For this review, take the finished solid that the model builds, in its own axes (mm). A direction names the side the tool comes from. Round coordinates to 2 decimals unless told otherwise and drop trailing zeros. Order: outer loops, then holes, each group sorted by start corner. A loop starts at its lowest first (then second) coordinate and runs counter-clockwise, first axis right, second up. Notation, with made-up numbers: (71.25, -36.75) -> (82.25, -36.75) arc R23 ccw to (82.25, -11.75) -> close; hole circle Ø1 at (31.25, -22.75). An arc over 180 degrees is marked (long way). Use a Markdown table: item, result. Add a question column.
1) Consider section C-C (x = 30). State the section outline as (y, z) points (3 decimals).
2) Consider section A-A (y = -7). State the section outline as (x, z) points (3 decimals), plus the area to 3 significant figures.
3) Clearance check with flat-ended pins moving along their axes: P1, Ø1.6, axis at y = 0.5, z = 11, coming from the +X side; P2, Ø1, axis at y = 1, z = 44, coming from the -X side; P3, Ø4, axis at x = 66.5, y = -5.5, coming from the -Z side (3 decimals). State where each tip first meets the part, or that it passes through.
4) Wall thickness on line 1 along Z through (x, y) = (30, 1) (3 decimals); line 2 along X through (y, z) = (-7.5, 26); line 3 along Y through (x, z) = (14, 24): over which ranges is each line inside the solid? List them lowest first. Write a range as [from, to].
5) Consider section D-D (y = 1). State the section outline as (x, z) points (3 decimals), plus the area to 3 significant figures.
6) Draft analysis for pull direction X (two halves, no side actions). For faces 5 (the face through (63.4, 1, 44)), 6 (the face through (-5, -3, 28)), 7 (the face through (60.4, 1, 45)), 8 (the face through (66, -9, 28)), state which applies: pulls with the +X half, pulls with the -X half, needs draft (parallel to the pull), parting line crosses it, or undercut.
7) Consider section B-B (z = 6). State the section outline as (x, y) points.
8) Machinability: for faces 1 (the face through (39, 0, 29)), 2 (the face through (63.4, 1, 13)), 3 (the face through (31, 1, 3)), 4 (the face through (-3, -3, 31.755)), which of the approach directions +Z, -Z, +X, -X, +Y, -Y give a long, thin tool a straight path to every point of the face, cutting with its end or side? Answer none if there is none.
```python
from build123d import *

# Parameters (mm, degrees)
SKETCH_1_W      = 57.4
SKETCH_1_H      = 19.255
SKETCH_1_H_2    = 21.645
EXTRUDE_1_DEPTH = 2
FILLET_1_R      = 2
SKETCH_2_W      = 4
SKETCH_2_H      = 7.5
EXTRUDE_2_DEPTH = 9


with BuildPart() as part:
    # Эскиз1 → Бобышка-Вытянуть1 (new body)
    with BuildSketch(Plane(origin=(0, 0, 0), x_dir=(1, 0, 0), z_dir=(0, 1, 0))):
        Polygon((63.4, -24.255), (68.4, -24.255), (68.4, -31.755), (63.4, -31.755), (63.4, -58.4), (0, -58.4), (0, -31.755), (-5, -31.755), (-5, -24.255), (0, -24.255), (0, 0), (63.4, 0), align=None)
        with Locations((31.7, -12.6275)):
            Rectangle(SKETCH_1_W, SKETCH_1_H, mode=Mode.SUBTRACT)
        with Locations((31.7, -44.5775)):
            Rectangle(SKETCH_1_W, SKETCH_1_H_2, mode=Mode.SUBTRACT)
    extrude(amount=EXTRUDE_1_DEPTH)

    # Скругление1
    fillet_1_edges = [part.edges().sort_by_distance(p)[0] for p in [
        (0, 1, 0),
        (63.4, 1, 0),
        (63.4, 1, 58.4),
        (0, 1, 58.4),
    ]]
    fillet(fillet_1_edges, radius=FILLET_1_R)

    # Эскиз2 → Бобышка-Вытянуть2 (add)
    with BuildSketch(Plane(origin=(0, 0, 0), x_dir=(-1, 0, 0), z_dir=(0, -1, 0))):
        with Locations((3, -28.005)):
            Rectangle(SKETCH_2_W, SKETCH_2_H)
        with Locations((-66.4, -28.005)):
            Rectangle(SKETCH_2_W, SKETCH_2_H)
    extrude(amount=EXTRUDE_2_DEPTH)


solid = part.part
```
Results list:
| question | item | result |
|---|---|---|
| 1 | outline | (0, 0) -> (2, 0) -> (2, 3) -> (0, 3) -> close; (0, 22.255) -> (2, 22.255) -> (2, 33.755) -> (0, 33.755) -> close; (0, 55.4) -> (2, 55.4) -> (2, 58.4) -> (0, 58.4) -> close |
| 2 | outline | (-5, 24.255) -> (-1, 24.255) -> (-1, 31.755) -> (-5, 31.755) -> close; (64.4, 24.255) -> (68.4, 24.255) -> (68.4, 31.755) -> (64.4, 31.755) -> close |
| 2 | area | 60.0 mm2 |
| 3 | P1 | x = 63.4 |
| 3 | P2 | x = 0 |
| 3 | P3 | z = 24.255 |
| 4 | line 1 | [0, 3], [22.255, 33.755], [55.4, 58.4] |
| 4 | line 2 | [-5, -1], [64.4, 68.4] |
| 4 | line 3 | [0, 2] |
| 5 | outline | (-5, 24.255) -> (0, 24.255) -> (0, 2) arc R2 ccw to (2, 0) -> (61.4, 0) arc R2 ccw to (63.4, 2) -> (63.4, 24.255) -> (68.4, 24.255) -> (68.4, 31.755) -> (63.4, 31.755) -> (63.4, 56.4) arc R2 ccw to (61.4, 58.4) -> (2, 58.4) arc R2 ccw to (0, 56.4) -> (0, 31.755) -> (-5, 31.755) -> close; hole (3, 3) -> (60.4, 3) -> (60.4, 22.255) -> (3, 22.255) -> close; hole (3, 33.755) -> (60.4, 33.755) -> (60.4, 55.4) -> (3, 55.4) -> close |
| 5 | area | 1,430 mm2 |
| 6 | face 5 | pulls with the +X half |
| 6 | face 6 | pulls with the -X half |
| 6 | face 7 | undercut |
| 6 | face 8 | needs draft |
| 7 | outline | (0, 0) -> (3, 0) -> (3, 2) -> (0, 2) -> close; (60.4, 0) -> (63.4, 0) -> (63.4, 2) -> (60.4, 2) -> close |
| 8 | face 1 | +Z, -Z, -Y |
| 8 | face 2 | -Z, +X, +Y, -Y |
| 8 | face 3 | +Y, -Y |
| 8 | face 4 | +Z, -X, +Y, -Y |
